Here's how the part is built. I have some questions about the finished solid (model axes, mm). Face numbers are marked on the shaded views. Round coordinates to 2 decimals unless told otherwise and drop trailing zeros. Write each loop counter-clockwise with the first axis right and the second up, starting at its lowest first coordinate (ties: lowest second). Pieces come first, ordered by that corner, then holes. Notation, with made-up numbers: M -23.75,-2 L 14.25,-2 A20 ccw 14.25,4 Z; hole C 81,-11 d5. An arc over 180 degrees is marked long. Write item = value, one per line. Start each with the question number.
(1) I want a section at A-A (y = 2.25). List the corners of the cut face in (x, z) for me.
(2) Will this pin go through, and if not, where does the flat tip stop? pin 1 Ø5 at (x, z) = (108.5, 3.5) entering from +Y.
(3) I need wall thicknesses on line 1 along Y through (x, z) = (-105, 7.5); line 2 along Y through (x, z) = (91, 5); line 3 along X through (y, z) = (23, 7). Which ranges of each line are inside material? Lowest first, please.
(4) I want a section at B-B (z = 6). Give the number of separate pieces and of enclosed holes in the cut face, and give its area (3 significant figures).
(5) If we mould it in two halves opening along Z, with no side actions, what happens to the marked faces 1 and 2? For each: released by +Z, released by -Z, zero draft, split by the parting line, or undercut.
(6) I want a section at C-C (y = 24). List the corners of the cut face in (x, z) for me, and give its area (3 significant figures).
```python
from build123d import *

# Parameters (mm, degrees)
SKETCH1_W           = 240
SKETCH1_H           = 60.5
SKETCH1_R           = 3.2
SKETCH1_R_2         = 1.5
BOSS_EXTRUDE1_DEPTH = 10
CUT_EXTRUDE1_DEPTH  = 11
CHAMFER3_SIZE       = 5


with BuildPart() as part:
    # Sketch1 → Boss-Extrude1 (new body)
    with BuildSketch(Plane.XY):
        Rectangle(SKETCH1_W, SKETCH1_H)
        with Locations((-105, 2.25)):
            Circle(SKETCH1_R, mode=Mode.SUBTRACT)
        with Locations((-105, -17.75)):
            Circle(SKETCH1_R, mode=Mode.SUBTRACT)
        with Locations((105, -17.75)):
            Circle(SKETCH1_R, mode=Mode.SUBTRACT)
        with Locations((105, 2.25)):
            Circle(SKETCH1_R, mode=Mode.SUBTRACT)
        with Locations((-91, 15.25)):
            Circle(SKETCH1_R_2, mode=Mode.SUBTRACT)
        with Locations((-79, 15.25)):
            Circle(SKETCH1_R_2, mode=Mode.SUBTRACT)
        with Locations((79, 15.25)):
            Circle(SKETCH1_R_2, mode=Mode.SUBTRACT)
        with Locations((91, 15.25)):
            Circle(SKETCH1_R_2, mode=Mode.SUBTRACT)
    extrude(amount=BOSS_EXTRUDE1_DEPTH)

    # Sketch2 → Cut-Extrude1 (cut, through all)
    with BuildSketch(Plane.XY.offset(10)):
        Polygon((-120, 14.25), (-105, 14.25), (-95, 30.25), (-120, 30.25), align=None)
        Polygon((120, 30.25), (120, 14.25), (105, 14.25), (95, 30.25), align=None)
    extrude(amount=-CUT_EXTRUDE1_DEPTH, mode=Mode.SUBTRACT)

    # Chamfer3
    chamfer3_edges = [part.edges().sort_by_distance(p)[0] for p in [
        (-120, 14.25, 5),
        (120, 14.25, 5),
        (120, -30.25, 5),
        (-120, -30.25, 5),
    ]]
    chamfer(chamfer3_edges, length=CHAMFER3_SIZE)


solid = part.part
```
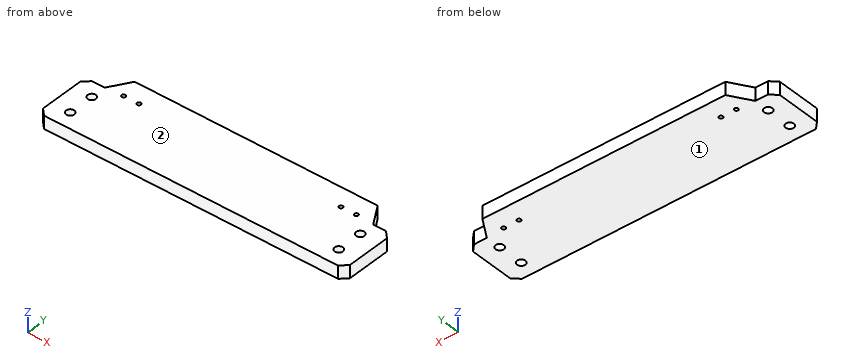
Returned:
q1.outline = M -120,0 L -108.2,0 L -108.2,10 L -120,10 Z; M -101.8,0 L 101.8,0 L 101.8,10 L -101.8,10 Z; M 108.2,0 L 120,0 L 120,10 L 108.2,10 Z
q2.pin_1 = 14.25
q3.line_1 = -30.25 to -20.95, -14.55 to -0.95, 5.45 to 14.25
q3.line_2 = -30.25 to 13.75, 16.75 to 30.25
q3.line_3 = -99.53 to 99.53
q4.separate_pieces = 1
q4.enclosed_holes = 8
q4.area = 13,700 mm²
q5.face_1 = released by -Z
q5.face_2 = released by +Z
q6.outline = M -98.91,0 L 98.91,0 L 98.91,10 L -98.91,10 Z
q6.area = 1,980 mm²
